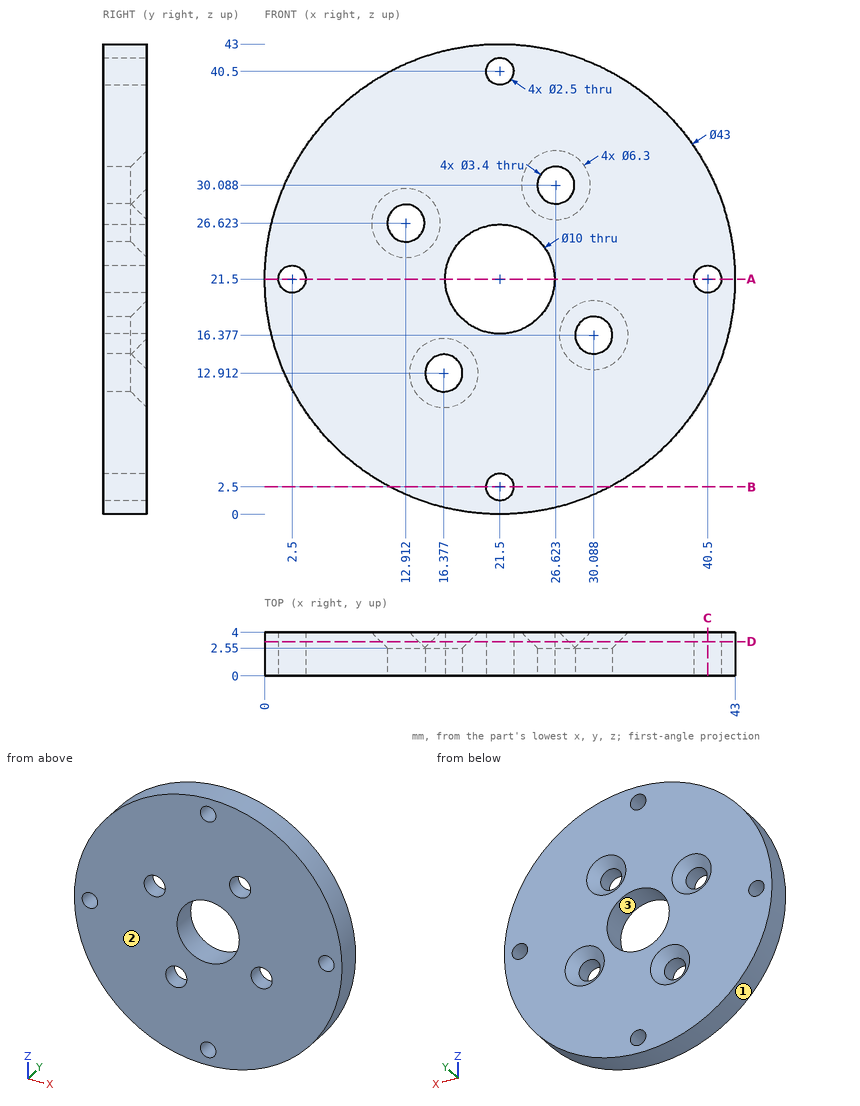
Can you work these out from the drawing? Everything is in mm from the part's minimum corner. Round coordinates to 2 decimals unless told otherwise and drop trailing zeros. Loops run counter-clockwise (first coordinate to the right, second up) from the corner with the lowest first, then second, coordinate; pieces in that order, holes last.
1. If we section it at D-D on y = 3.15: Count the separate pieces of the cut face and the enclosed holes in it, plus the area to 3 significant figures.
Answer list:
separate pieces: 1
enclosed holes: 9
area: 1,290 mm2
2. If we section it at A-A on z = 21.5: Write out the boundary of the cut face in (x, y), plus the area to 3 significant figures.
Answer list:
outline: (0, 0) - (1.25, 0) - (1.25, 4) - (0, 4) - close; (3.75, 0) - (16.5, 0) - (16.5, 4) - (3.75, 4) - close; (26.5, 0) - (39.25, 0) - (39.25, 4) - (26.5, 4) - close; (41.75, 0) - (43, 0) - (43, 4) - (41.75, 4) - close
area: 112 mm2
3. We'd pull the mould along Z, two halves only. Please class the marked faces 1, 2 and 3: +Z half, -Z half, draft (parallel to the pull), parting line (faces both ways), or undercut.
Answer list:
face 1: parting line
face 2: draft
face 3: undercut
4. For P1, Ø1.5, axis at x = 37, y = 3, coming from the +Z side; P2, Ø4.5, axis at x = 30.09, z = 16.38, coming from the +Y side (1 decimal); P3, Ø1.5, axis at y = 1, z = 5.5, coming from the -X side (1 decimal); P4, Ø1.5, axis at x = 40.5, z = 21.5, coming from the +Y side, each with a flat end and sliding along its axis, tell me the tip position at first contact or that it passes through.
Answer list:
P1: stops at z = 37.14
P2: stops at y = 3.1
P3: stops at x = 6.3
P4: passes through
5. If we section it at B-B on z = 2.5: Write out the boundary of the cut face in (x, y).
Answer list:
outline: (11.44, 0) - (20.25, 0) - (20.25, 4) - (11.44, 4) - close; (22.75, 0) - (31.56, 0) - (31.56, 4) - (22.75, 4) - close
6. If we section it at C-C on x = 40.5: Write out the boundary of the cut face in (y, z), plus the area to 3 significant figures.
Answer list:
outline: (0, 11.44) - (4, 11.44) - (4, 20.25) - (0, 20.25) - close; (0, 22.75) - (4, 22.75) - (4, 31.56) - (0, 31.56) - close
area: 70.5 mm2
7. If I drill on line 1 along X through (y, z) = (2.75, 21.5); line 2 along X through (y, z) = (3.8, 28) (1 decimal); line 3 along X through (y, z) = (3.8, 27.5) (1 decimal), over which ranges is the centre line in solid material (lowest first)?
Answer list:
line 1: x = 0 to 1.25, 3.75 to 16.5, 26.5 to 39.25, 41.75 to 43
line 2: x = 1 to 10.3, 15.5 to 24.5, 28.7 to 42
line 3: x = 0.9 to 10.1, 15.7 to 25.2, 28 to 42.1
